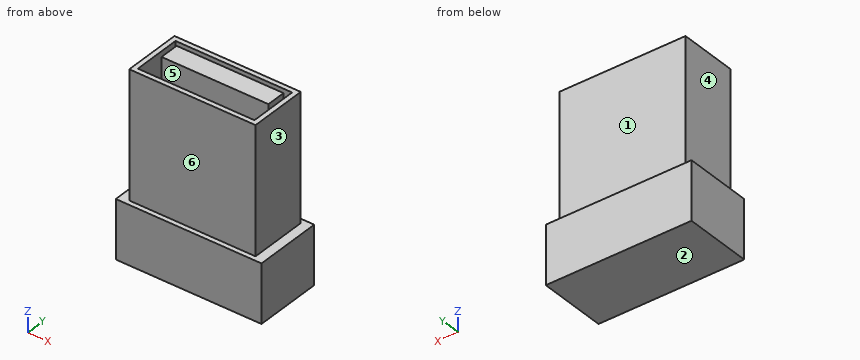
```python
from build123d import *

# Parameters (mm, degrees)
SKETCH_1_W          = 13
SKETCH_1_H          = 5
SKETCH_1_W_2        = 6
SKETCH_1_H_2        = 7
EXTRUDE_1_DEPTH     = 6
SKETCH_3_W          = 6
SKETCH_3_H          = 7
EXTRUDE_2_DEPTH     = 7.5
SKETCH_4_W          = 12
SKETCH_4_H          = 5
SKETCH_4_W_2        = 11
SKETCH_4_H_2        = 2
CUT_EXTRUDE_1_DEPTH = 13
SKETCH_5_W          = 13
SKETCH_5_H          = 6
SKETCH_5_W_2        = 12
SKETCH_5_H_2        = 5
EXTRUDE_1_2_DEPTH   = 13


with BuildPart() as part:
    # 草图1 → Extrude 1 (new body, symmetric)
    with BuildSketch(Plane(origin=(0, 0, 0), x_dir=(0, 0, -1), z_dir=(1, 0, 0))):
        with Locations((-6.5, 2.5)):
            Rectangle(SKETCH_1_W, SKETCH_1_H)
        with Locations((3, 2.5)):
            Rectangle(SKETCH_1_W_2, SKETCH_1_H_2)
    extrude(amount=EXTRUDE_1_DEPTH, both=True)

    # 草图3 → 凸台-拉伸2 (add, symmetric)
    with BuildSketch(Plane(origin=(0, 0, 0), x_dir=(0, 0, -1), z_dir=(1, 0, 0))):
        with Locations((3, 2.5)):
            Rectangle(SKETCH_3_W, SKETCH_3_H)
    extrude(amount=EXTRUDE_2_DEPTH, both=True)

    # 草图4 → 切除-拉伸1 (cut)
    with BuildSketch(Plane.XY.offset(13)):
        with Locations((0, 2.5)):
            Rectangle(SKETCH_4_W, SKETCH_4_H)
        with Locations((0, 3.5)):
            Rectangle(SKETCH_4_W_2, SKETCH_4_H_2, mode=Mode.SUBTRACT)
    extrude(amount=-CUT_EXTRUDE_1_DEPTH, mode=Mode.SUBTRACT)

    # 草图5 → Extrude 1 2 (add)
    with BuildSketch(Plane.XY):
        with Locations((0, 2.5)):
            Rectangle(SKETCH_5_W, SKETCH_5_H)
        with Locations((0, 2.5)):
            Rectangle(SKETCH_5_W_2, SKETCH_5_H_2, mode=Mode.SUBTRACT)
    extrude(amount=EXTRUDE_1_2_DEPTH)


solid = part.part
```
Model file for the job. Use its own axes, mm. Face numbers are marked on the shaded views. A direction names the side the tool comes from. Round coordinates to 2 decimals unless told otherwise and drop trailing zeros. Write each loop counter-clockwise with the first axis right and the second up, starting at its lowest first coordinate (ties: lowest second). Pieces come first, ordered by that corner, then holes. Notation, with made-up numbers: (-38, 21.25) - (-33, 21.25) arc R23 ccw to (-33, 36.25) - close; hole circle Ø1 at (34, 54). An arc over 180 degrees is marked (long way). One line per item, written item: value.
(1) Cut at A-A, the plane z = 11.5. Give the cut face in (x, y).
Values follow:
outline: (-6.5, -0.5) - (6.5, -0.5) - (6.5, 5.5) - (-6.5, 5.5) - close; (-5.5, 2.5) - (5.5, 2.5) - (5.5, 4.5) - (-5.5, 4.5) - close; hole (-6, 0) - (6, 0) - (6, 5) - (-6, 5) - close
(2) Cut at C-C, the plane y = 0.25. Give the cut face in (x, z).
Values follow:
outline: (-7.5, -6) - (7.5, -6) - (7.5, 0) - (6.5, 0) - (6.5, 13) - (6, 13) - (6, 0) - (-6, 0) - (-6, 13) - (-6.5, 13) - (-6.5, 0) - (-7.5, 0) - close
(3) Wall check: probe 1 along Y at (x, z) = (3.5, 10.5); probe 2 along X at (y, z) = (3, 8.5); probe 3 along X at (y, z) = (0.5, 9.5). Give the ranges that are in metal, low to high.
Values follow:
probe 1: y = -0.5 to 0, 2.5 to 4.5, 5 to 5.5
probe 2: x = -6.5 to -6, -5.5 to 5.5, 6 to 6.5
probe 3: x = -6.5 to -6, 6 to 6.5
(4) Two-plate mould, pull along Y, no slides. Class the marked faces 4, 5 and 6: pulls with the +Y half, pulls with the -Y half, needs draft (parallel to the pull), parting line crosses it, or undercut.
Values follow:
face 4: needs draft
face 5: undercut
face 6: pulls with the -Y half
(5) Cut at D-D, the plane x = -1.75. Give the cut face in (y, z), plus the area to 3 significant figures.
Values follow:
outline: (-1, -6) - (6, -6) - (6, 0) - (5.5, 0) - (5.5, 13) - (5, 13) - (5, 0) - (4.5, 0) - (4.5, 13) - (2.5, 13) - (2.5, 0) - (0, 0) - (0, 13) - (-0.5, 13) - (-0.5, 0) - (-1, 0) - close
area: 81.0 mm²
(6) Drop flat-ended pins along their axis: P1, Ø1.5, axis at y = 2, z = 4, coming from the +X side; P2, Ø5.5, axis at x = -2.5, z = 6, coming from the +Y side; P3, Ø5.5, axis at x = -2.5, z = 7.5, coming from the -Y side. Give the stop position or say it passes through.
Values follow:
P1: stops at x = 6.5
P2: stops at y = 5.5
P3: stops at y = -0.5
(7) Cut at B-B, the plane x = 6.25. Give the cut face in (y, z).
Values follow:
outline: (-1, -6) - (6, -6) - (6, 0) - (5.5, 0) - (5.5, 13) - (-0.5, 13) - (-0.5, 0) - (-1, 0) - close
(8) 3-axis set-ups, long thin cutter, end or side, ignore diameter. For the marked faces 1, 2 and 3: which of +Z, -Z, +X, -X, +Y, -Y reach the whole face in a straight line?
Values follow:
face 1: +Z, +X, -X, +Y
face 2: -Z, +X, -X, +Y, -Y
face 3: +Z, +X, +Y, -Y
